The listing builds one solid part. Answer for the finished solid, in the listing's coordinates (mm). A direction names the side the tool comes from. Coordinates: 2 decimals unless noted, no trailing zeros. Order: outer loops, then holes, each group sorted by start corner. A loop starts at its lowest first (then second) coordinate and runs counter-clockwise, first axis right, second up.
Autodesk Inventor part; units mm, degrees
ref_plane "Work Plane1" through (0, 0, 7.5) normal (0, 0, 1) x (1, 0, 0)
ref_plane "YZ Plane" through (0, 0, 0) normal (1, 0, 0) x (0, 1, 0)
ref_plane "XZ Plane" through (0, 0, 0) normal (0, 1, 0) x (-1, 0, 0)
sketch "Sketch1" plane through (0, 0, 0) normal (0, 0, 1) x (1, 0, 0)
  line L0 (0, 0) -> (20.25, 0)
  line L1 (20.25, 0) -> (20.25, 40.5)
  line L2 (20.25, 40.5) -> (0, 40.5)
  line L3 (0, 40.5) -> (0, 0)
  dimension "d0" = 40.5
  dimension "d1" = 20.25
extrude "Extrusion1" add sketch "Sketch1" along normal blind 15
sketch "Sketch2" plane through (0, 0, 15) normal (0, 0, 1) x (1, 0, 0)
  line L0 (3.5, 37) -> (20.25, 37)
  line L1 (20.25, 37) -> (20.25, 3.5)
  line L2 (20.25, 3.5) -> (3.5, 3.5)
  line L3 (3.5, 3.5) -> (3.5, 37)
  line L4 (20.25, 0) -> (20.25, 40.5)
  line L5 (20.25, 40.5) -> (0, 40.5)
  line L6 (0, 0) -> (20.25, 0)
  dimension "d4" = 16.75
  dimension "d5" = 3.5
  dimension "d6" = 3.5
extrude "Extrusion2" cut sketch "Sketch2" against normal blind 15
ref_plane "Work Plane1" through (0, 0, 7.5) normal (0, 0, 1) x (1, 0, 0)
sketch "Sketch3" plane through (0, 0, 7.5) normal (0, 0, 1) x (1, 0, 0)
  line L0 (2.5, 38) -> (20.25, 38)
  line L1 (20.25, 38) -> (20.25, 2.5)
  line L2 (20.25, 2.5) -> (2.5, 2.5)
  line L3 (2.5, 2.5) -> (2.5, 38)
  line L4 (20.25, 0) -> (20.25, 3.5)
  line L5 (20.25, 40.5) -> (0, 40.5)
  line L6 (0, 0) -> (20.25, 0)
  line L7 (0, 40.5) -> (0, 0)
  dimension "d10" = 2.5
  dimension "d11" = 2.5
  dimension "d12" = 2.5
extrude "Extrusion3" cut sketch "Sketch3" along normal mid plane 5
sketch "Sketch4" plane through (20.25, 40.5, 15) normal (1, 0, 0) x (0, 0, -1)
  line L0 (15, 0) -> (0, 0)
  line L1 (0, 0) -> (15, 0)
  line L2 (15, 0) -> (15, 5)
  line L3 (15, 5) -> (0, 5)
  line L4 (0, 5) -> (0, 0)
  line L5 (15, -40.5) -> (15, -37)
  line L6 (15, -40.5) -> (0, -40.5)
  line L7 (0, -40.5) -> (0, -45.5)
  line L8 (0, -45.5) -> (15, -45.5)
  line L9 (15, -45.5) -> (15, -40.5)
  dimension "d15" = 5
  dimension "d16" = 5
extrude "Extrusion4" add sketch "Sketch4" against normal blind 20.25
sketch "Sketch5" plane through (0, 0, 15) normal (0, 0, 1) x (1, 0, 0)
  point P0 (0, 0)
sketch "Sketch6" plane through (20.25, 37, 10) normal (1, 0, 0) x (0, 0, -1)
  circle A0 centre (2.5, 4.5) radius 2.5
  circle A1 centre (2.5, -38) radius 2.5
  line L0 (10, 0) -> (10, 8.5)
  line L1 (0, 1) -> (5, 1)
  line L2 (10, 8.5) -> (-5, 8.5)
  line L3 (5, -34.5) -> (0, -34.5)
  point P0 (10, -37)
  dimension "d19" = 7.5
  dimension "d20" = 0
  dimension "d21" = 3.5
  dimension "d22" = 7.5
  dimension "d23" = 3.5
  dimension "d24" = 5
extrude "Extrusion5" cut sketch "Sketch6" against normal blind 50
sketch "Sketch7" plane through (0, 0, 15) normal (0, 0, 1) x (1, 0, 0)
  point P0 (0, 0)
sketch "Sketch8" plane through (0, 0, 15) normal (0, 0, 1) x (1, 0, 0)
  line L0 (20.25, 3.5) -> (20.25, -5)
  line L1 (10.25, 45.5) -> (20.25, 45.5)
  line L2 (20.25, 45.5) -> (20.25, -5)
  line L3 (20.25, -5) -> (10.25, -5)
  line L4 (10.25, -5) -> (10.25, 45.5)
  point P0 (0, 0)
  dimension "d27" = 10
extrude "Extrusion6" cut sketch "Sketch8" against normal through all
properties part number "standlower"
(1) Given pin 1 Ø4 at (y, z) = (13, 2) entering from +X; pin 2 Ø4 at (y, z) = (29, 7.5) entering from +X, each flat-ended and moving along its own axis, determine where each tip first touches the part or whether it passes through.
(2) Find section C-C on z = 5.5. Determine the outline of the cut face in (x, y), then the cut area to 3 significant figures.
(3) Find section A-A on x = 8.25. Determine the outline of the cut face in (y, z), then the cut area to 3 significant figures.
(4) A tool of negligible diameter and unlimited length cuts with its end or side. For faces 1 (the flat face through (3, 20, 5)), 2 (the flat face through (7, 3.5, 13)), 3 (the flat face through (5, -5, 8)), from which of +Z, -Z, +X, -X, +Y, -Y can it reach the whole face along a straight path? Write none if from no direction.
(5) Find section B-B on y = -1. Determine the outline of the cut face in (x, z), then the cut area to 4 significant figures.
(6) Find the intervals of material crossed by probe 1 along Y at (x, z) = (7.25, 7.5); probe 2 along Y at (x, z) = (7.5, 3.75); probe 3 along Y at (x, z) = (8, 6), in increasing order.
(7) Find section D-D on y = 32.5. Determine the outline of the cut face in (x, z).
(8) The mould has two halves that part along Z. Classify faces 4 (the flat face through (3, 21, 0)), 5 (the flat face through (3.5, 20, 3)), 6 (the cylindrical face through (5, -1, 10)): pulls with the +Z half, pulls with the -Z half, needs draft (parallel to the pull), parting line crosses it, or undercut.
Resolved:
1. pin 1: stops at x = 3.5
1. pin 2: stops at x = 2.5
2. outline: (0, -5) - (10.25, -5) - (10.25, -2.5) - (0, -2.5) - close; (0, 0.5) - (10.25, 0.5) - (10.25, 2.5) - (2.5, 2.5) - (2.5, 38) - (10.25, 38) - (10.25, 40) - (0, 40) - close; (0, 43) - (10.25, 43) - (10.25, 45.5) - (0, 45.5) - close
2. area: 181 mm2
3. outline: (-5, 0) - (3.5, 0) - (3.5, 5) - (2.5, 5) - (2.5, 10) - (3.5, 10) - (3.5, 15) - (-5, 15) - close; (37, 0) - (45.5, 0) - (45.5, 15) - (37, 15) - (37, 10) - (38, 10) - (38, 5) - (37, 5) - close; hole circle Ø5 at (-1, 7.5); hole circle Ø5 at (41.5, 7.5)
3. area: 206 mm2
4. face 1: +X
4. face 2: +Z, -Z, +X
4. face 3: +Z, -Z, +X, -X, -Y
5. outline: (0, 0) - (10.25, 0) - (10.25, 5) - (0, 5) - close; (0, 10) - (10.25, 10) - (10.25, 15) - (0, 15) - close
5. area: 102.5 mm2
6. probe 1: y = -5 to -3.5, 1.5 to 2.5, 38 to 39, 44 to 45.5
6. probe 2: y = -5 to 3.5, 37 to 45.5
6. probe 3: y = -5 to -3, 1 to 2.5, 38 to 39.5, 43.5 to 45.5
7. outline: (0, 0) - (3.5, 0) - (3.5, 5) - (2.5, 5) - (2.5, 10) - (3.5, 10) - (3.5, 15) - (0, 15) - close
8. face 4: pulls with the -Z half
8. face 5: needs draft
8. face 6: undercut
